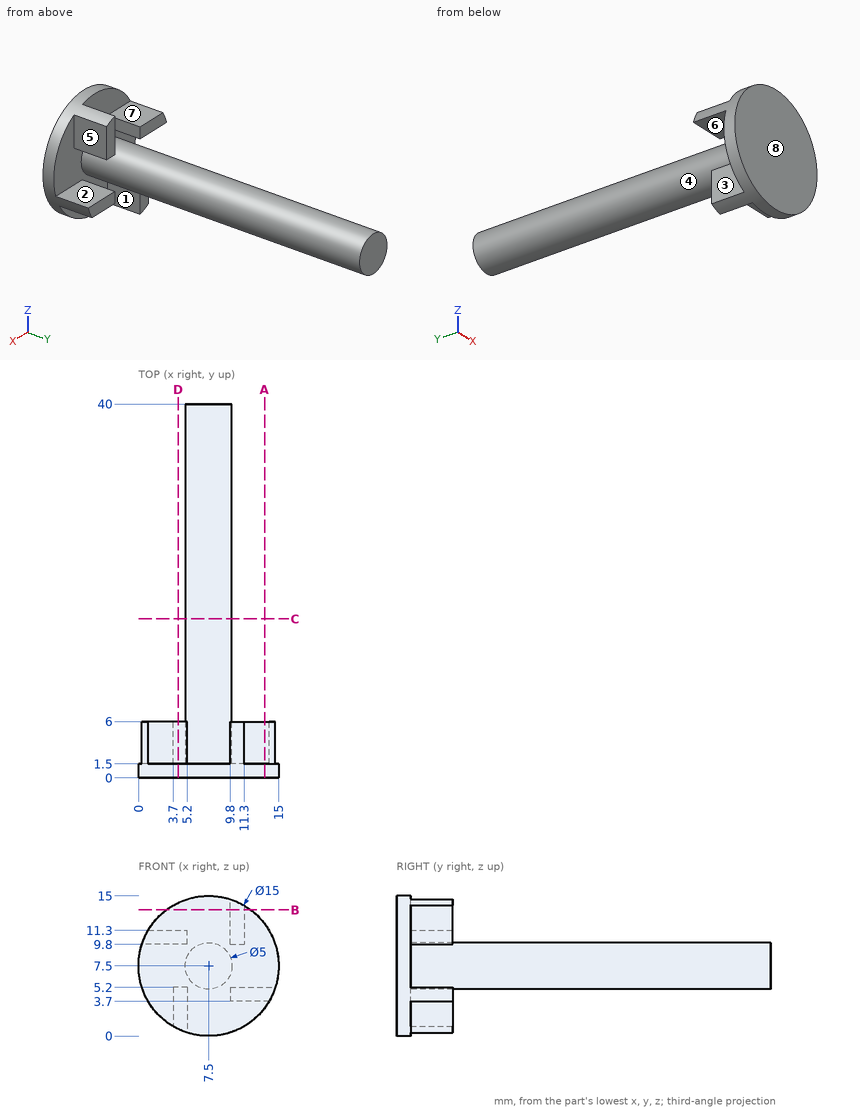
Drawing for the job (mm, zero at the part's lowest x, y, z). A direction names the side the tool comes from. Give positions to 0.01 mm unless a question says otherwise; leave off trailing zeros. Loops run counter-clockwise (first coordinate to the right, second up) from the corner with the lowest first, then second, coordinate; pieces in that order, holes last.
(1) 3-axis set-ups, long thin cutter, end or side, ignore diameter. For the marked faces 1, 2, 3, 4 and 5: which of +Z, -Z, +X, -X, +Y, -Y reach the whole face in a straight line?
Return value:
face 1: -Z, +Y
face 2: +X, +Y
face 3: -Z, -X, +Y
face 4: +Y
face 5: +Z, +X, +Y
(2) Pull direction Z, two halves, no side cores. Call the marked faces 6, 7 and 8: pulls with the +Z half, pulls with the -Z half, needs draft (parallel to the pull), parting line crosses it, or undercut.
Return value:
face 6: undercut
face 7: pulls with the +Z half
face 8: needs draft
(3) Band-saw the part on B-B (z = 13.5). Write the cut outline in (x, y).
Return value:
outline: (3, 0) - (12, 0) - (12, 1.5) - (11.3, 1.5) - (11.3, 6) - (9.8, 6) - (9.8, 1.5) - (3, 1.5) - close
(4) Band-saw the part on D-D (x = 4.25). Write the cut outline in (y, z), and give its area (3 significant figures).
Return value:
outline: (0, 0.74) - (6, 0.74) - (6, 5.2) - (1.5, 5.2) - (1.5, 9.8) - (6, 9.8) - (6, 11.3) - (1.5, 11.3) - (1.5, 14.26) - (0, 14.26) - close
area: 47.1 mm2
(5) Band-saw the part on C-C (y = 17). Write the cut outline in (x, z).
Return value:
outline: circle Ø5 at (7.5, 7.5)
(6) Band-saw the part on A-A (x = 13.5). Write the cut outline in (y, z).
Return value:
outline: (0, 3) - (1.5, 3) - (1.5, 3.7) - (6, 3.7) - (6, 5.2) - (1.5, 5.2) - (1.5, 12) - (0, 12) - close
(7) Drill centre lines: line 1 along Y through (x, z) = (5.5, 1.5); line 2 along X through (y, z) = (18, 8.5). Where is each one in solid material? Low to high.
Return value:
line 1: y = 0 to 1.5
line 2: x = 5.21 to 9.79
(8) Pin check, flat tips, straight feed: pin 1 (5 mm diameter, centred on x = 4, y = 18.5, fed in from -Z); pin 2 (5 mm diameter, centred on x = 7.5, z = 13, fed in from +Y); pin 3 (1.2 mm diameter, centred on x = 10.5, y = 3, fed in from -Z); pin 4 (1.5 mm diameter, centred on x = 11.5, y = 11, fed in from +Z). Stop position of each tip, or through.
Return value:
pin 1: stops at z = 5.21
pin 2: stops at y = 6
pin 3: stops at z = 3.7
pin 4: passes through
